The listing builds one solid part. Answer for the finished solid, in the listing's coordinates (mm). A direction names the side the tool comes from. Coordinates: 2 decimals unless noted, no trailing zeros. Order: outer loops, then holes, each group sorted by start corner. A loop starts at its lowest first (then second) coordinate and runs counter-clockwise, first axis right, second up.
```python
from build123d import *

# Parameters (mm, degrees)
CYLINDER032_R                = 9.5
CYLINDER032_DEPTH            = 27
CYLINDER035_R                = 23
CYLINDER035_DEPTH            = 5
CYLINDER046_R                = 2.2
CYLINDER046_DEPTH            = 5
ARRAY022_Y_COUNT             = 2
ARRAY022_Y_PITCH             = 57
BOX_W                        = 10.4
BOX_H                        = 57
BOX_DEPTH                    = 5
CYLINDER048_R                = 5.2
CYLINDER048_DEPTH            = 5
ARRAY021_Y_COUNT             = 2
ARRAY021_Y_PITCH             = 57
CUT002004004_PLACEMENT_ANGLE = 305
BOX008_W                     = 56
BOX008_H                     = 3
BOX008_DEPTH                 = 3
FILLET004_R                  = 1.6
CYLINDER031_R                = 12.5
CYLINDER031_DEPTH            = 27
FILLET_R                     = 2
CYLINDER030_R                = 1.95
CYLINDER030_DEPTH            = 5
ARRAY015_X_COUNT             = 2
ARRAY015_X_PITCH             = 70
BOX004_W                     = 70
BOX004_H                     = 12
BOX004_DEPTH                 = 5
CYLINDER029_R                = 6
CYLINDER029_DEPTH            = 5
ARRAY014_X_COUNT             = 2
ARRAY014_X_PITCH             = 70
FUSION018_PLACEMENT_ANGLE    = 55


with BuildPart() as zero_holder_internal_cylinder:
    # Cylinder032 → Cylinder032 (new body)
    with BuildSketch(Plane.XY):
        Circle(CYLINDER032_R)
    extrude(amount=CYLINDER032_DEPTH)


with BuildPart() as zero_holder_top_disk:
    # Cylinder035 → Cylinder035 (new body)
    with BuildSketch(Plane.XY.offset(22)):
        Circle(CYLINDER035_R)
    extrude(amount=CYLINDER035_DEPTH)


with BuildPart() as extract_fusion:
    # Cylinder046 → Cylinder046 (new body)
    with BuildSketch(Plane.XY):
        Circle(CYLINDER046_R)
    extrude(amount=CYLINDER046_DEPTH)

    # Array022 Y: extract fusion ×2


with BuildPart() as extract_fusion_1:
    add(extract_fusion.part)
    with Locations(*[(0, i * ARRAY022_Y_PITCH, 0) for i in range(1, ARRAY022_Y_COUNT)]):
        add(extract_fusion.part)


with BuildPart() as extract_fusion_2:
    # Array022 placement: moved
    add(extract_fusion_1.part.moved(Location((0, -28.5, 0))))


with BuildPart() as between_hole_cube:
    # Box → Box (new body)
    with BuildSketch(Plane(origin=(-5.2, -28.5, 0), x_dir=(1, 0, 0), z_dir=(0, 0, 1))):
        with Locations((5.2, 28.5)):
            Rectangle(BOX_W, BOX_H)
    extrude(amount=BOX_DEPTH)


with BuildPart() as microscope_attachment_cut:
    # Cylinder048 → Cylinder048 (new body)
    with BuildSketch(Plane.XY):
        Circle(CYLINDER048_R)
    extrude(amount=CYLINDER048_DEPTH)

    # Array021 Y: microscope attachment cut ×2


with BuildPart() as microscope_attachment_cut_1:
    add(microscope_attachment_cut.part)
    with Locations(*[(0, i * ARRAY021_Y_PITCH, 0) for i in range(1, ARRAY021_Y_COUNT)]):
        add(microscope_attachment_cut.part)


with BuildPart() as microscope_attachment_cut_2:
    # Array021 placement: moved
    add(microscope_attachment_cut_1.part.moved(Location((0, -28.5, 0))))

    # Fusion023: union between hole cube
    add(between_hole_cube.part)

    # Cut002004004: cut extract fusion
    add(extract_fusion_2.part, mode=Mode.SUBTRACT)


with BuildPart() as microscope_attachment_cut_3:
    # Cut002004004 placement: moved
    add(microscope_attachment_cut_2.part.moved(Location((0, 0, 22))).rotate(Axis((0, 0, 22), (0, 0, 1)), CUT002004004_PLACEMENT_ANGLE))


with BuildPart() as sprint_plate_fillet:
    # Box008 → Box008 (new body)
    with BuildSketch(Plane(origin=(-28, -1.5, 19), x_dir=(1, 0, 0), z_dir=(0, 0, 1))):
        with Locations((28, 1.5)):
            Rectangle(BOX008_W, BOX008_H)
    extrude(amount=BOX008_DEPTH)

    # Fillet004
    fillet004_edges = [sprint_plate_fillet.edges().sort_by_distance(p)[0] for p in [
        (-28, 0, 19),
        (28, 0, 19),
    ]]
    fillet(fillet004_edges, radius=FILLET004_R)


with BuildPart() as zero_holder_external_cylinder_fillet:
    # Cylinder031 → Cylinder031 (new body)
    with BuildSketch(Plane.XY):
        Circle(CYLINDER031_R)
    extrude(amount=CYLINDER031_DEPTH)

    # Fillet
    fillet_edges = [zero_holder_external_cylinder_fillet.edges().sort_by_distance(p)[0] for p in [
        (-12.5, 0, 0),
    ]]
    fillet(fillet_edges, radius=FILLET_R)


with BuildPart() as spring_plate_end_array003:
    # Cylinder030 → Cylinder030 (new body)
    with BuildSketch(Plane.XY):
        Circle(CYLINDER030_R)
    extrude(amount=CYLINDER030_DEPTH)

    # Array015 X: spring plate end array003 ×2


with BuildPart() as spring_plate_end_array003_1:
    add(spring_plate_end_array003.part)
    with Locations(*[(i * ARRAY015_X_PITCH, 0, 0) for i in range(1, ARRAY015_X_COUNT)]):
        add(spring_plate_end_array003.part)


with BuildPart() as cube:
    # Box004 → Box004 (new body)
    with BuildSketch(Plane(origin=(0, -6, 0), x_dir=(1, 0, 0), z_dir=(0, 0, 1))):
        with Locations((35, 6)):
            Rectangle(BOX004_W, BOX004_H)
    extrude(amount=BOX004_DEPTH)


with BuildPart() as zero_holder_cut:
    # Cylinder029 → Cylinder029 (new body)
    with BuildSketch(Plane.XY):
        Circle(CYLINDER029_R)
    extrude(amount=CYLINDER029_DEPTH)

    # Array014 X: zero holder cut ×2


with BuildPart() as zero_holder_cut_1:
    add(zero_holder_cut.part)
    with Locations(*[(i * ARRAY014_X_PITCH, 0, 0) for i in range(1, ARRAY014_X_COUNT)]):
        add(zero_holder_cut.part)

    # Fusion017: union Cube
    add(cube.part)

    # Cut010: cut spring plate end array003
    add(spring_plate_end_array003_1.part, mode=Mode.SUBTRACT)


with BuildPart() as zero_holder_cut_2:
    # Cut010 placement: moved
    add(zero_holder_cut_1.part.moved(Location((-35, 0, 22))))

    # Fusion018: union zero holder top disk, microscope attachment cut, sprint plate fillet, zero holder external cylinder fillet
    add(zero_holder_top_disk.part)
    add(microscope_attachment_cut_3.part)
    add(sprint_plate_fillet.part)
    add(zero_holder_external_cylinder_fillet.part)


with BuildPart() as zero_holder_cut_3:
    # Fusion018 placement: moved
    add(zero_holder_cut_2.part.rotate(Axis((0, 0, 0), (0, 0, 1)), FUSION018_PLACEMENT_ANGLE))

    # Cut011: cut zero holder internal cylinder
    add(zero_holder_internal_cylinder.part, mode=Mode.SUBTRACT)


solid = zero_holder_cut_3.part
```
(1) For faces 1 (the face through (10.545, 6.713, 11.86)), 2 (the face through (11.44, 26.8, 24.46)), 3 (the face through (-21.4, -20.1, 24.5)), 4 (the face through (-16.04, -22.95, 21.29)), determine the directions among +Z, -Z, +X, -X, +Y, -Y from which every point of the face is accessible in a straight line to the end or side of a thin tool.
(2) Find section B-B (y = 0). Write down the section's boundary in (x, z), and give its area (3 significant figures).
(3) The mould has two halves that part along X. Classify faces 5 (the face through (-11.54, -26.94, 24.46)), 6 (the face through (16.08, 22.92, 21.29)), 7 (the face through (0, -10, 0)): released by +X, released by -X, zero draft, split by the parting line, or undercut.
(4) Find section D-D (z = 19.75). Write down the section's boundary in (x, y), and give its area (3 significant figures).
(5) Each of these flat-tipped pins is pushed along its axis until it touches: pin 1 Ø3 at (x, y) = (8.5, 15.5) entering from -Z; pin 2 Ø1.5 at (y, z) = (25, 24.5) entering from -X; pin 3 Ø2 at (x, z) = (-7.5, 11.5) entering from -Y. Where does it stop, or does it pass through?
(6) Consider line 1 (Y direction, x = 0, z = 23.3); line 2 (Y direction, x = 0, z = 8.25); line 3 (Z direction, x = 20.5, y = 22). Determine where each line is inside the solid, lowest interval first.
(7) Find section A-A (x = 0). Write down the section's boundary in (y, z).
(8) Find section C-C (z = 23.75). Write down the section's boundary in (x, y), and give its area (3 significant figures).
Findings below:
1. face 1: -Z
1. face 2: +Z, -Z, +Y
1. face 3: +Z, -Z, -X
1. face 4: -Z, -X, -Y
2. outline: (-23, 22) - (-12.5, 22) - (-12.5, 2) arc R2 ccw to (-10.5, 0) - (-9.5, 0) - (-9.5, 27) - (-23, 27) - close; (9.5, 0) - (10.5, 0) arc R2 ccw to (12.5, 2) - (12.5, 22) - (23, 22) - (23, 27) - (9.5, 27) - close
2. area: 265 mm2
3. face 5: undercut
3. face 6: released by +X
3. face 7: zero draft
4. outline: (-17.15, -21.88) - (-14.69, -23.6) - (-5.89, -11.03) arc R12.5 ccw to (8.35, 9.31) - (17.15, 21.88) - (14.69, 23.6) - (5.89, 11.03) arc R12.5 ccw to (-8.35, -9.31) - close; hole circle Ø19 at (0, 0)
4. area: 299 mm2
5. pin 1: stops at z = 19
5. pin 2: stops at x = -5.2
5. pin 3: stops at y = -10.68
6. line 1: y = -33.7 to -30.7, -26.3 to -9.5, 9.5 to 26.3, 30.7 to 33.7
6. line 2: y = -12.5 to -9.5, 9.5 to 12.5
6. line 3: z = 22 to 27
7. outline: (-33.7, 22) - (-30.7, 22) - (-30.7, 27) - (-33.7, 27) - close; (-26.3, 22) - (-12.5, 22) - (-12.5, 2) arc R2 ccw to (-10.5, 0) - (-9.5, 0) - (-9.5, 27) - (-26.3, 27) - close; (9.5, 0) - (10.5, 0) arc R2 ccw to (12.5, 2) - (12.5, 22) - (26.3, 22) - (26.3, 27) - (9.5, 27) - close; (30.7, 22) - (33.7, 22) - (33.7, 27) - (30.7, 27) - close
8. outline: (-24.99, -25.23) arc R6 ccw to (-15.16, -32.11) - (-7.82, -21.63) arc R23 ccw to (-5.2, -22.4) - (-5.2, -28.5) arc R5.2 ccw to (5.2, -28.5) - (5.2, -22.4) arc R23 ccw to (17.65, 14.75) - (24.99, 25.23) arc R6 ccw to (15.16, 32.11) - (7.82, 21.63) arc R23 ccw to (5.2, 22.4) - (5.2, 28.5) arc R5.2 ccw to (-5.2, 28.5) - (-5.2, 22.4) arc R23 ccw to (-17.65, -14.75) - close; hole circle Ø3.9 at (-20.08, -28.67); hole circle Ø19 at (0, 0); hole circle Ø4.4 at (0, -28.5); hole circle Ø4.4 at (0, 28.5); hole circle Ø3.9 at (20.08, 28.67)
8. area: 1,930 mm2
